```python
from build123d import *

# Parameters (mm, degrees)
SKETCH2_W           = 71
SKETCH2_H           = 47.6
SKETCH2_R           = 3.35
SKETCH2_R_2         = 1
SKETCH2_W_2         = 10.344
SKETCH2_H_2         = 3.1
BOSS_EXTRUDE1_DEPTH = 3


with BuildPart() as part:
    # Sketch2 → Boss-Extrude1 (new body)
    with BuildSketch(Plane(origin=(0, 0, 0), x_dir=(1, 0, 0), z_dir=(0, 1, 0))):
        with Locations((35.5, 23.8)):
            Rectangle(SKETCH2_W, SKETCH2_H)
        with Locations((35.5, 20.9)):
            Circle(SKETCH2_R, mode=Mode.SUBTRACT)
        with Locations((43, 20.9)):
            Circle(SKETCH2_R_2, mode=Mode.SUBTRACT)
        with Locations((49, 20.9)):
            Circle(SKETCH2_R_2, mode=Mode.SUBTRACT)
        with Locations((39.25, 14.404809472)):
            Circle(SKETCH2_R_2, mode=Mode.SUBTRACT)
        with Locations((42.25, 9.208657049)):
            Circle(SKETCH2_R_2, mode=Mode.SUBTRACT)
        with Locations((31.75, 14.404809472)):
            Circle(SKETCH2_R_2, mode=Mode.SUBTRACT)
        with Locations((28.75, 9.208657049)):
            Circle(SKETCH2_R_2, mode=Mode.SUBTRACT)
        with Locations((28, 20.9)):
            Circle(SKETCH2_R_2, mode=Mode.SUBTRACT)
        with Locations((22, 20.9)):
            Circle(SKETCH2_R_2, mode=Mode.SUBTRACT)
        with Locations((31.75, 27.395190528)):
            Circle(SKETCH2_R_2, mode=Mode.SUBTRACT)
        with Locations((28.75, 32.591342951)):
            Circle(SKETCH2_R_2, mode=Mode.SUBTRACT)
        with Locations((39.25, 27.395190528)):
            Circle(SKETCH2_R_2, mode=Mode.SUBTRACT)
        with Locations((42.25, 32.591342951)):
            Circle(SKETCH2_R_2, mode=Mode.SUBTRACT)
        with Locations((10.684, 42.95)):
            Rectangle(SKETCH2_W_2, SKETCH2_H_2, mode=Mode.SUBTRACT)
        with Locations((27.228, 42.95)):
            Rectangle(SKETCH2_W_2, SKETCH2_H_2, mode=Mode.SUBTRACT)
        with Locations((43.772, 42.95)):
            Rectangle(SKETCH2_W_2, SKETCH2_H_2, mode=Mode.SUBTRACT)
        with Locations((60.316, 42.95)):
            Rectangle(SKETCH2_W_2, SKETCH2_H_2, mode=Mode.SUBTRACT)
    extrude(amount=BOSS_EXTRUDE1_DEPTH)


solid = part.part
```
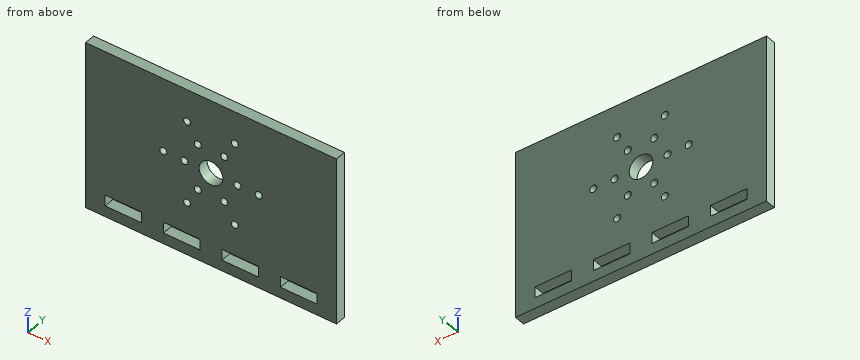
Can you work these out from the model? Positions are in its coordinate system, mm. Coordinates: 2 decimals unless noted, no trailing zeros. Loops run counter-clockwise (first coordinate to the right, second up) from the corner with the lowest first, then second, coordinate; pieces in that order, holes last. Notation, with made-up numbers: (77.5, 18.25) -> (83.5, 18.25) arc R19 cw to (83.5, 48.25) -> close; hole circle Ø2 at (52.5, 8.25). An arc over 180 degrees is marked (long way). Put each result on its own line as item: value. Start each with the question number.
Q1. I want a section at A-A (x = 45). Write out the boundary of the cut face in (y, z).
Q2. I'm going to push flat-ended pins straight in: P1, Ø1.5, axis at x = 27.5, y = 2, coming from the +Z side; P2, Ø1.8, axis at x = 22, z = -20.9, coming from the -Y side. Where does each tip first touch, or does it pass through?
Q3. If I drill on line 1 (Z direction, x = 31.75, y = 1.4); line 2 (X direction, y = 1.2, z = -20.9); line 3 (Z direction, x = 55.5, y = 1.65), over which ranges is the centre line in solid material (lowest first)? Write a range as [from, to].
Q4. I want a section at B-B (x = 35.5). Write out the boundary of the cut face in (y, z), plus the area to 3 significant figures.
Q5. I want a section at C-C (y = 2.4). Count the separate pieces of the cut face and the enclosed holes in it, plus the area to 3 significant figures.
Taken from the geometry:
1. outline: (0, -47.6) -> (3, -47.6) -> (3, -44.5) -> (0, -44.5) -> close; (0, -41.4) -> (3, -41.4) -> (3, 0) -> (0, 0) -> close
2. P1: stops at z = 0
2. P2: passes through
3. line 1: z = [-47.6, -44.5], [-41.4, -28.4], [-26.4, -15.4], [-13.4, 0]
3. line 2: x = [0, 21], [23, 27], [29, 32.15], [38.85, 42], [44, 48], [50, 71]
3. line 3: z = [-47.6, -44.5], [-41.4, 0]
4. outline: (0, -47.6) -> (3, -47.6) -> (3, -24.25) -> (0, -24.25) -> close; (0, -17.55) -> (3, -17.55) -> (3, 0) -> (0, 0) -> close
4. area: 123 mm2
5. separate pieces: 1
5. enclosed holes: 17
5. area: 3,180 mm2
